```python
from build123d import *

# Parameters (mm, degrees)
F1_DEPTH = 40
F2_SIZE  = 2.5
F3_R     = 1.5


with BuildPart() as f1:
    # F0 (on Top) → F1 (new body)
    with BuildSketch(Plane.XY):
        with BuildLine():
            Line((0, -3), (0, 0))
            Line((0, 0), (0, 18))
            Line((0, 18), (0, 41))
            Line((0, 41), (-28, 41))
            Line((-28, 41), (-28, 38))
            Line((-28, 38), (-3, 38))
            Line((-3, 38), (-3, 18))
            Line((-3, 18), (-52.5, 18))
            ThreePointArc((-52.5, 18), (-56.035534, 16.535534), (-57.5, 13))
            Line((-57.5, 13), (-57.5, -3))
            Line((-57.5, -3), (-53, -3))
            Line((-53, -3), (-44.5, -3))
            Line((-44.5, -3), (-44.5, 0))
            Line((-44.5, 0), (-44.5, 2))
            Line((-44.5, 2), (-46.5, 2))
            Line((-46.5, 2), (-46.5, 0))
            Line((-46.5, 0), (-54.5, 0))
            Line((-54.5, 0), (-54.5, 10))
            ThreePointArc((-54.5, 10), (-53.035534, 13.535534), (-49.5, 15))
            Line((-49.5, 15), (-3, 15))
            Line((-3, 15), (-3, 0))
            Line((-3, 0), (-9, 0))
            Line((-9, 0), (-9, 2))
            Line((-9, 2), (-11, 2))
            Line((-11, 2), (-11, 0))
            Line((-11, 0), (-11, -3))
            Line((-11, -3), (0, -3))
        make_face()
    extrude(amount=F1_DEPTH)

    # F2
    f2_edges = [f1.edges().sort_by_distance(p)[0] for p in [
        (-11, -3, 20),
        (-44.5, -3, 20),
    ]]
    chamfer(f2_edges, length=F2_SIZE)

    # F3
    f3_edges = [f1.edges().sort_by_distance(p)[0] for p in [
        (-3, 18, 20),
        (-3, 38, 20),
    ]]
    fillet(f3_edges, radius=F3_R)


solid = f1.part
```
The listing builds one solid part. Answer for the finished solid, in the listing's coordinates (mm). A direction names the side the tool comes from. Coordinates: 2 decimals unless noted, no trailing zeros. Loops run counter-clockwise (first coordinate to the right, second up) from the corner with the lowest first, then second, coordinate; pieces in that order, holes last. Notation, with made-up numbers: M -20.5,-26.5 L 1.5,-26.5 A15 cw 1.5,-22.5 Z; hole C 88.5,10.5 d11. An arc over 180 degrees is marked long. Answer as a JSON object with one key per item and string values. Group by question number.
Item 1: Section D-D (z = 7) is taken. Write down the section's boundary in (x, y), and give its area (3 significant figures).
Item 2: Section B-B (y = 3) is taken. Write down the section's boundary in (x, z), and give its area (3 significant figures).
Item 3: Consider L1, parallel to X at y = 1, z = 37.5; L2, parallel to Y at x = -4.5, z = 8.5; L3, parallel to X at y = 8.5, z = 13.5. Determine where each line is inside the solid, lowest interval first.
Item 4: Section A-A (x = -15.5) is taken. Write down the section's boundary in (y, z), and give its area (3 significant figures).
Item 5: Section C-C (x = -6.5) is taken. Write down the section's boundary in (y, z).
Item 6: Determine the mould class of faces 1 (the face through (-46.5, 1, 20)), 2 (the face through (-28, 40, 20)), 3 (the face through (-50, 0, 20)), 4 (the face through (-9.7, -1.8, 19.7)) for opening direction Y: +Y half, -Y half, draft (parallel to the pull), parting line (faces both ways), or undercut.
Item 7: Each of these flat-tipped pins is pushed along its axis until it touches: P1, Ø12, axis at y = 19, z = 14, coming from the +X side; P2, Ø3.5, axis at y = 39, z = 12.5, coming from the -X side; P3, Ø5, axis at y = 31.5, z = 24.5, coming from the -X side; P4, Ø6, axis at y = 18, z = 5, coming from the -X side. Where does it stop, or does it pass through?
Item 8: Which of the six approach directions +Z, -Z, +X, -X, +Y, -Y give full straight-line access (tool end or side, diameter ignored) to faces 5 (the face through (-10, 2, 20)), 6 (the face through (-11, 1, 20)), 7 (the face through (-16, 38, 20))?
Solved:
{
 "1": {"outline": "M -57.5,-3 L -47,-3 L -44.5,-0.5 L -44.5,2 L -46.5,2 L -46.5,0 L -54.5,0 L -54.5,10 A5 cw -49.5,15 L -3,15 L -3,0 L -9,0 L -9,2 L -11,2 L -11,-0.5 L -8.5,-3 L 0,-3 L 0,41 L -28,41 L -28,38 L -4.5,38 A1.5 cw -3,36.5 L -3,19.5 A1.5 cw -4.5,18 L -52.5,18 A5 ccw -57.5,13 Z", "area": "481 mm2"},
 "2": {"outline": "M -57.5,0 L -54.5,0 L -54.5,40 L -57.5,40 Z; M -3,0 L 0,0 L 0,40 L -3,40 Z", "area": "240 mm2"},
 "3": {"L1": "x = -57.5 to -54.5, -46.5 to -44.5, -11 to -9, -3 to 0", "L2": "y = -3 to 0, 15 to 18, 38 to 41", "L3": "x = -57.5 to -54.5, -3 to 0"},
 "4": {"outline": "M 15,0 L 18,0 L 18,40 L 15,40 Z; M 38,0 L 41,0 L 41,40 L 38,40 Z", "area": "240 mm2"},
 "5": {"outline": "M -3,0 L 0,0 L 0,40 L -3,40 Z; M 15,0 L 18,0 L 18,40 L 15,40 Z; M 38,0 L 41,0 L 41,40 L 38,40 Z"},
 "6": {"face 1": "undercut", "face 2": "draft", "face 3": "undercut", "face 4": "-Y half"},
 "7": {"P1": "stops at x = 0", "P2": "stops at x = -28", "P3": "stops at x = -3", "P4": "stops at x = -57.08"},
 "8": {"face 5": "+Z, -Z", "face 6": "+Z, -Z, -Y", "face 7": "+Z, -Z, -X"}
}
